Can you work these out from the model? Positions are in its coordinate system, mm. A direction names the side the tool comes from. Coordinates: 2 decimals unless noted, no trailing zeros. Order: outer loops, then holes, each group sorted by start corner. A loop starts at its lowest first (then second) coordinate and runs counter-clockwise, first axis right, second up. Notation, with made-up numbers: (36.5, 80.25) -> (93.5, 80.25) arc R31 cw to (93.5, 116.25) -> close; hole circle Ø5 at (44, -28). An arc over 180 degrees is marked (long way). Use a Markdown table: item, result. Add a question column.
1. For faces 4 (the cylindrical face through (9.094, 1.085, -6.368)), 5 (the flat face through (0, 3.5, 0)), 6 (the flat face through (-12.5, 2, -7)), which set-ups out of +Z, -Z, +X, -X, +Y, -Y let a thin tool reach every point of the face, with its end or its side?
2. Suppose I cut it at A-A, the plane y = 4.6. List the corners of the cut face in (x, z) for me.
3. We'd pull the mould along Z, two halves only. Please class faces 1 (the flat face through (0, 4, -8.8)), 2 (the flat face through (-1, 0, 0)), 3 (the flat face through (-13.486, 2.465, -2.768)): pulls with the +Z half, pulls with the -Z half, needs draft (parallel to the pull), parting line crosses it, or undercut.
4. For pin 1 Ø10 at (x, z) = (2.5, 1.5) entering from +Y; pin 2 Ø2 at (y, z) = (1.5, -6.5) entering from -X; pin 3 Ø0.9 at (x, z) = (8.5, -7.5) entering from -Y, each with a flat end and sliding along its axis, tell me the tip position at first contact or that it passes through.
5. Suppose I cut it at C-C, the plane z = 7.8. List the corners of the cut face in (x, y) for me, then the cut area to 3 significant figures.
6. If I drill on line 1 along X through (y, z) = (0.95, 7.8); line 2 along Z through (x, y) = (4.75, 4.05); line 3 along Z through (x, y) = (8, 2), over which ranges is the centre line in solid material (lowest first)? Write a range as from..to.
7. Suppose I cut it at D-D, the plane x = -6. List the corners of the cut face in (y, z) for me, then the cut area to 3 significant figures.
8. Suppose I cut it at B-B, the plane y = 1.25. List the corners of the cut face in (x, z) for me.
```python
from build123d import *

# Parameters (mm, degrees)
RESSALTO_EXTRUS_O1_DEPTH = 3.5
ESBO_O1_3_W              = 25
ESBO_O1_3_H              = 2
ESBO_O1_3_W_2            = 2
ESBO_O1_3_H_2            = 3
RESSALTO_EXTRUS_O2_DEPTH = 5
ESBO_O2_R                = 1.55
CORTE_EXTRUS_O1_DEPTH    = 2.2


with BuildPart() as part:
    # Esbo_o1 → Ressalto-extrus_o1 (new body)
    with BuildSketch(Plane(origin=(0, 0, 0), x_dir=(1, 0, 0), z_dir=(0, 1, 0))):
        Polygon((12.5, -8.8), (12.5, 8.8), (-12.5, 8.8), (-12.5, 4), (-12.5, 1.5), (-12.5, -1.5), (-12.5, -4), (-12.5, -8.8), align=None)
    extrude(amount=RESSALTO_EXTRUS_O1_DEPTH)

    # Esbo_o1_3 → Ressalto-extrus_o2 (add)
    with BuildSketch(Plane(origin=(0, 0, 0), x_dir=(1, 0, 0), z_dir=(0, 1, 0))):
        with Locations((0, -9.8)):
            Rectangle(ESBO_O1_3_W, ESBO_O1_3_H)
        with Locations((0, 9.8)):
            Rectangle(ESBO_O1_3_W, ESBO_O1_3_H)
        Polygon((-12.5, 1.5), (-12.5, 4), (-14.5, 1.5), align=None)
        with Locations((-13.5, 0)):
            Rectangle(ESBO_O1_3_W_2, ESBO_O1_3_H_2)
        Polygon((-14.5, -1.5), (-12.5, -4), (-12.5, -1.5), align=None)
    extrude(amount=RESSALTO_EXTRUS_O2_DEPTH)

    # Esbo_o2 → Corte-extrus_o1 (cut)
    with BuildSketch(Plane.XZ):
        with Locations(Location((8.5, 7.8, 0), (0, 0, 270))):
            Circle(ESBO_O2_R)
        with Locations(Location((-8.5, 7.8, 0), (0, 0, 90))):
            Circle(ESBO_O2_R)
        with Locations(Location((-8.5, -7.8, 0), (0, 0, 270))):
            Circle(ESBO_O2_R)
        with Locations(Location((8.5, -7.8, 0), (0, 0, 90))):
            Circle(ESBO_O2_R)
    extrude(amount=-CORTE_EXTRUS_O1_DEPTH, mode=Mode.SUBTRACT)


solid = part.part
```
Worked out:
| question | item | result |
|---|---|---|
| 1 | face 4 | -Y |
| 1 | face 5 | +X, +Y |
| 1 | face 6 | -Z, -X, +Y, -Y |
| 2 | outline | (-14.5, -1.5) -> (-12.5, -4) -> (-12.5, 4) -> (-14.5, 1.5) -> close; (-12.5, -10.8) -> (12.5, -10.8) -> (12.5, -8.8) -> (-12.5, -8.8) -> close; (-12.5, 8.8) -> (12.5, 8.8) -> (12.5, 10.8) -> (-12.5, 10.8) -> close |
| 3 | face 1 | undercut |
| 3 | face 2 | needs draft |
| 3 | face 3 | pulls with the -Z half |
| 4 | pin 1 | stops at y = 3.5 |
| 4 | pin 2 | stops at x = -12.5 |
| 4 | pin 3 | stops at y = 2.2 |
| 5 | outline | (-12.5, 0) -> (-10.05, 0) -> (-10.05, 2.2) -> (-6.95, 2.2) -> (-6.95, 0) -> (6.95, 0) -> (6.95, 2.2) -> (10.05, 2.2) -> (10.05, 0) -> (12.5, 0) -> (12.5, 3.5) -> (-12.5, 3.5) -> close |
| 5 | area | 73.9 mm² |
| 6 | line 1 | x = -12.5..-10.05, -6.95..6.95, 10.05..12.5 |
| 6 | line 2 | z = -10.8..-8.8, 8.8..10.8 |
| 6 | line 3 | z = -10.8..-9.27, -6.33..6.33, 9.27..10.8 |
| 7 | outline | (0, -10.8) -> (5, -10.8) -> (5, -8.8) -> (3.5, -8.8) -> (3.5, 8.8) -> (5, 8.8) -> (5, 10.8) -> (0, 10.8) -> close |
| 7 | area | 81.6 mm² |
| 8 | outline | (-14.5, -1.5) -> (-12.5, -4) -> (-12.5, -10.8) -> (12.5, -10.8) -> (12.5, 10.8) -> (-12.5, 10.8) -> (-12.5, 4) -> (-14.5, 1.5) -> close; hole circle Ø3.1 at (-8.5, -7.8); hole circle Ø3.1 at (-8.5, 7.8); hole circle Ø3.1 at (8.5, -7.8); hole circle Ø3.1 at (8.5, 7.8) |
